```python
from build123d import *

# Parameters (mm, degrees)
SKETCH1_W           = 74.93
SKETCH1_H           = 144.907
SKETCH1_W_2         = 55.88
SKETCH1_H_2         = 4.191
SKETCH1_W_3         = 49.53
SKETCH1_H_3         = 104.775
BOSS_EXTRUDE1_DEPTH = 3.175


with BuildPart() as part:
    # Sketch1 → Boss-Extrude1 (new body)
    with BuildSketch(Plane(origin=(0, 0, 0), x_dir=(1, 0, 0), z_dir=(0, 1, 0))):
        Rectangle(SKETCH1_W, SKETCH1_H)
        with Locations((0, -64.008)):
            Rectangle(SKETCH1_W_2, SKETCH1_H_2, mode=Mode.SUBTRACT)
        with Locations((0, 64.008)):
            Rectangle(SKETCH1_W_2, SKETCH1_H_2, mode=Mode.SUBTRACT)
        Rectangle(SKETCH1_W_3, SKETCH1_H_3, mode=Mode.SUBTRACT)
    extrude(amount=BOSS_EXTRUDE1_DEPTH)


solid = part.part
```
Source: CAD feature listing. Evaluate the final solid. Frame: model axes, mm. A direction names the side the tool comes from. Coordinates: 2 decimals unless noted, no trailing zeros. Loops run counter-clockwise (first coordinate to the right, second up) from the corner with the lowest first, then second, coordinate; pieces in that order, holes last. Notation, with made-up numbers: M 39,58.5 L 75,58.5 A6 ccw 75,62.5 Z; hole C 2.25,14.25 d3. An arc over 180 degrees is marked long. Use CSV: the item, a comma, the result in double quotes.
(1) Cut plane C-C on y = 1.85. Return loops of the section in (x, z) (1 decimal).
Answers follow:
outline,"M -37.5,-72.5 L 37.5,-72.5 L 37.5,72.5 L -37.5,72.5 Z; hole M -27.9,-66.1 L 27.9,-66.1 L 27.9,-61.9 L -27.9,-61.9 Z; hole M -27.9,61.9 L 27.9,61.9 L 27.9,66.1 L -27.9,66.1 Z; hole M -24.8,-52.4 L 24.8,-52.4 L 24.8,52.4 L -24.8,52.4 Z"
(2) Cut plane B-B on x = -19. Return loops of the section in (y, z) (1 decimal), and give its area (3 significant figures).
Answers follow:
outline,"M 0,-72.5 L 3.2,-72.5 L 3.2,-66.1 L 0,-66.1 Z; M 0,-61.9 L 3.2,-61.9 L 3.2,-52.4 L 0,-52.4 Z; M 0,52.4 L 3.2,52.4 L 3.2,61.9 L 0,61.9 Z; M 0,66.1 L 3.2,66.1 L 3.2,72.5 L 0,72.5 Z"
area,"101 mm²"
(3) Draft query along X for faces 1 (the face through (37.465, 2, 1)), 2 (the face through (0, 2, -52.388)), 3 (the face through (-25, 3.175, 0)). Return one class per face: pulls with the +X half, pulls with the -X half, needs draft (parallel to the pull), parting line crosses it, or undercut.
Answers follow:
face 1,"pulls with the +X half"
face 2,"undercut"
face 3,"needs draft"
(4) Cut plane A-A on z = -1.5. Return loops of the section in (x, y) (3 decimals), and give its area (3 significant figures).
Answers follow:
outline,"M -37.465,0 L -24.765,0 L -24.765,3.175 L -37.465,3.175 Z; M 24.765,0 L 37.465,0 L 37.465,3.175 L 24.765,3.175 Z"
area,"80.6 mm²"
(5) Reachability of faces 4 (the face through (-1, 2, 72.454)), 5 (the face through (-24.765, 2, 1)) from +Z, -Z, +X, -X, +Y, -Y: full face, straight path, thin tool, end or side. Return the list, or none.
Answers follow:
face 4,"+Z, +X, -X, +Y, -Y"
face 5,"+Y, -Y"
(6) Line query: line 1 (Z direction, x = -14, y = 1.6); line 2 (X direction, y = 0.85, z = 17) (3 decimals); line 3 (X direction, y = 2.5, z = -62.5) (3 decimals). Output: solid intervals per line, ascending. Write a range as [from, to].
Answers follow:
line 1,"[-72.45, -66.1], [-61.91, -52.39], [52.39, 61.91], [66.1, 72.45]"
line 2,"[-37.465, -24.765], [24.765, 37.465]"
line 3,"[-37.465, -27.94], [27.94, 37.465]"
